from build123d import *

# Parameters (mm, degrees)
CUT_EXTRUDE2_DEPTH = 4


# Read off the part's stored shape, not the designer's step: CSK for M2 Flat Head Machine Screw1
with BuildPart() as part:
    # Sketch1 → Revolve1 (revolve)
    with BuildSketch(Plane.XY, mode=Mode.PRIVATE) as revolve1_sk:
        Polygon((54, 11), (55.5, 11), (55.5, -4), (48, -4), (48, -3), (54, -3), align=None)
    revolve(revolve1_sk.sketch.rotate(Axis((0, 0, 0), (0, 1, 0)), 90), axis=Axis((0, 0, 0), (0, 1, 0)))

    # Sketch7 → Cut-Extrude2 (cut)
    with BuildSketch(Plane(origin=(0, 11, 0), x_dir=(1, 0, 0), z_dir=(0, 1, 0))):
        with BuildLine():
            Line((-17.150443188, -52.783636654), (-16.686917696, -51.35705188))
            ThreePointArc((-16.686917696, -51.35705188), (-27, -46.765371804), (-36.133052743, -40.129820576))
            Line((-36.133052743, -40.129820576), (-37.136748653, -41.244537814))
            ThreePointArc((-37.136748653, -41.244537814), (-27.75, -48.06440991), (-17.150443188, -52.783636654))
        make_face()
    extrude(amount=-CUT_EXTRUDE2_DEPTH, mode=Mode.SUBTRACT)

    # CSK for M2 Flat Head Machine Screw1 outl → CSK for M2 Flat Head Machine Screw1 (revolve, cut)
    with BuildSketch(Plane(origin=(0, 0, 0), x_dir=(0, 1, 0), z_dir=(-0.121869343405148, 0, -0.992546151641322))):
        Polygon((2.200019656, 55.500019656), (0, 55.500019656), (0, 53.986657854), (1.2, 53.986657854), (1.2, 54.5), align=None)
    revolve(axis=Axis((0, 0, 0), (0.992546151641322, 0, -0.121869343405148)), mode=Mode.SUBTRACT)

    # CSK for M2 Flat Head Machine Screw1 2 ou → CSK for M2 Flat Head Machine Screw1 2 (revolve, cut)
    with BuildSketch(Plane(origin=(0, 0, 0), x_dir=(0, 1, 0), z_dir=(0.12186934340514702, 0, -0.9925461516413221))):
        Polygon((2.200023885, 55.500023885), (0, 55.500023885), (0, 53.986657854), (1.2, 53.986657854), (1.2, 54.5), align=None)
    revolve(axis=Axis((0, 0, 0), (0.9925461516413221, 0, 0.12186934340514702)), mode=Mode.SUBTRACT)

    # CSK for M2 Flat Head Machine Screw1 3 ou → CSK for M2 Flat Head Machine Screw1 3 (revolve, cut)
    with BuildSketch(Plane(origin=(0, 0, 0), x_dir=(0.9205048534524387, 0, -0.3907311284892778), z_dir=(0, -1, 0))):
        Polygon((0, -55.500018568), (2.200018568, -55.500018568), (1.2, -54.5), (1.2, -53.986657854), (0, -53.986657854), align=None)
    revolve(axis=Axis((0, 0, 0), (0.3907311284892778, 0, 0.9205048534524387)), mode=Mode.SUBTRACT)

    # CSK for M2 Flat Head Machine Screw1 4 ou → CSK for M2 Flat Head Machine Screw1 4 (revolve, cut)
    with BuildSketch(Plane(origin=(0, 0, 0), x_dir=(0.79863551004729, 0, -0.601815023152052), z_dir=(0, -1, 0))):
        Polygon((0, -55.500012206), (2.200012206, -55.500012206), (1.2, -54.5), (1.2, -53.986657854), (0, -53.986657854), align=None)
    revolve(axis=Axis((0, 0, 0), (0.601815023152052, 0, 0.79863551004729)), mode=Mode.SUBTRACT)

    # CSK for M2 Flat Head Machine Screw1 5 ou → CSK for M2 Flat Head Machine Screw1 5 (revolve, cut)
    with BuildSketch(Plane(origin=(0, 0, 0), x_dir=(0.9205048534524416, 0, 0.39073112848927083), z_dir=(0, 1, 0))):
        Polygon((0, -55.500018348), (2.200018348, -55.500018348), (1.2, -54.5), (1.2, -53.986657854), (0, -53.986657854), align=None)
    revolve(axis=Axis((0, 0, 0), (0.39073112848927083, 0, -0.9205048534524416)), mode=Mode.SUBTRACT)

    # CSK for M2 Flat Head Machine Screw1 6 ou → CSK for M2 Flat Head Machine Screw1 6 (revolve, cut)
    with BuildSketch(Plane(origin=(0, 0, 0), x_dir=(0.7986355100472992, 0, 0.60181502315204), z_dir=(0, 1, 0))):
        Polygon((0, -55.50002414), (2.20002414, -55.50002414), (1.2, -54.5), (1.2, -53.986657854), (0, -53.986657854), align=None)
    revolve(axis=Axis((0, 0, 0), (0.60181502315204, 0, -0.7986355100472992)), mode=Mode.SUBTRACT)


solid = part.part
Read the model definition and answer for the solid it produces. Units are mm, in the model's axes. A direction names the side the tool comes from. Coordinates: 2 decimals unless noted, no trailing zeros. Order: outer loops, then holes, each group sorted by start corner. A loop starts at its lowest first (then second) coordinate and runs counter-clockwise, first axis right, second up. Notation, with made-up numbers: M 86,33.5 L 119,33.5 A29 ccw 119,62.5 Z; hole C 57,-39.75 d8. An arc over 180 degrees is marked long. Put each result on its own line as item: value. Start each with the question number.
Item 1: Section B-B, the plane z = 0 is taken. Determine the outline of the cut face in (x, y).
Item 2: Section C-C, the plane y = 4.5 is taken. Determine the outline of the cut face in (x, z), plus the area to 3 significant figures.
Item 3: Given pin 1 Ø1.5 at (y, z) = (3.5, -0.5) entering from +X; pin 2 Ø6.5 at (x, z) = (-30, 48) entering from +Y; pin 3 Ø8 at (x, y) = (-23.5, 3) entering from +Z, each flat-ended and moving along its own axis, determine where each tip first touches the part or whether it passes through.
Item 4: The mould has two halves that part along Y. Classify faces 1 (the face through (-14.418, -3.493, -45.783)), 2 (the face through (-20.139, -0.36, 50.375)), 3 (the face through (53.7, -0.16, 7.79)), 4 (the face through (-27, 7, 47)): +Y half, -Y half, draft (parallel to the pull), parting line (faces both ways), or undercut.
Item 5: For faces 5 (the face through (-16.671, 3.395, -52.937)), 6 (the face through (32, -3, -36)), determine the directions among +Z, -Z, +X, -X, +Y, -Y from which every point of the face is accessible in a straight line to the end or side of a thin tool.
Item 6: Consider probe 1 along X at (y, z) = (4.5, 0); probe 2 along X at (y, z) = (9, -44.5); probe 3 along Y at (x, z) = (14.5, -46). Determine where each line is inside the solid, lowest interval first. Write a range as [from, to].
Item 7: Section A-A, the plane x = 0 is taken. Determine the outline of the cut face in (y, z).
Computed:
1. outline: M -55.5,-4 L -48,-4 L -48,-3 L -54,-3 L -54,11 L -55.5,11 Z; M 48,-4 L 55.5,-4 L 55.5,11 L 54,11 L 54,-3 L 48,-3 Z
2. outline: C 0,0 d111; hole C 0,0 d108
2. area: 516 mm2
3. pin 1: stops at x = 55.5
3. pin 2: stops at y = 7
3. pin 3: stops at z = 51.96
4. face 1: draft
4. face 2: undercut
4. face 3: undercut
4. face 4: +Y half
5. face 5: +Y, -Y
5. face 6: +Y
6. probe 1: x = [-55.5, -54], [54, 55.5]
6. probe 2: x = [-33.17, -30.59], [30.59, 33.17]
6. probe 3: y = [-4, -3]
7. outline: M -4,-55.5 L 11,-55.5 L 11,-54 L -3,-54 L -3,-48 L -4,-48 Z; M -4,48 L -3,48 L -3,54 L 11,54 L 11,55.5 L -4,55.5 Z
